Build history of the part. All positions in model axes, mm. Face numbers are marked on the shaded views. A direction names the side the tool comes from. Round coordinates to 2 decimals unless told otherwise and drop trailing zeros. Write each loop counter-clockwise with the first axis right and the second up, starting at its lowest first coordinate (ties: lowest second). Pieces come first, ordered by that corner, then holes. Notation, with made-up numbers: (-3.5, 19) -> (34.5, 19) arc R33 cw to (34.5, 58) -> close; hole circle Ø4 at (65.5, 49.5). An arc over 180 degrees is marked (long way). Answer as CSV lines item,"result".
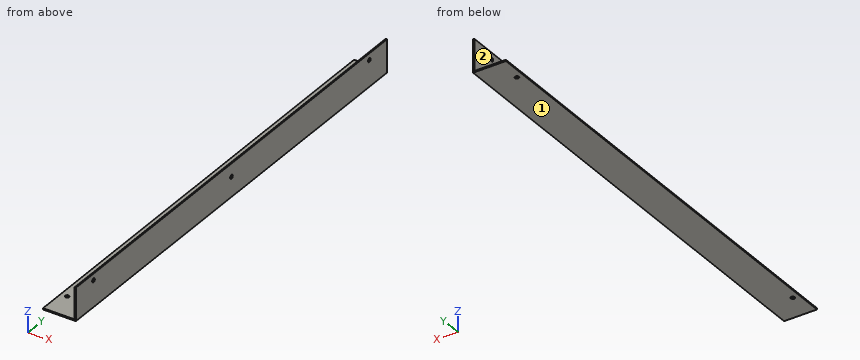
from build123d import *

# Parameters (mm, degrees)
CROQUIS2_W              = 1
CROQUIS2_H              = 354
SALIENTE_EXTRUIR2_DEPTH = 25
CROQUIS5_R              = 1.5
CORTAR_EXTRUIR2_DEPTH   = 1
CROQUIS1_W              = 24
CROQUIS1_H              = 354
CROQUIS1_R              = 1.5
SALIENTE_EXTRUIR3_DEPTH = 1


with BuildPart() as part:
    # Croquis2 → Saliente-Extruir2 (new body)
    with BuildSketch(Plane.XY):
        with Locations((-55.758230402, -111.819349421)):
            Rectangle(CROQUIS2_W, CROQUIS2_H)
    extrude(amount=SALIENTE_EXTRUIR2_DEPTH)

    # Croquis5 → Cortar-Extruir2 (cut)
    with BuildSketch(Plane(origin=(-55.258230402, 0, 0), x_dir=(0, 0, -1), z_dir=(1, 0, 0))):
        with Locations((-20, 45.180650579)):
            Circle(CROQUIS5_R)
        with Locations((-20, -268.819349421)):
            Circle(CROQUIS5_R)
        with Locations((-15, -111.819349421)):
            Circle(CROQUIS5_R)
    extrude(amount=-CORTAR_EXTRUIR2_DEPTH, mode=Mode.SUBTRACT)

    # Croquis1 → Saliente-Extruir3 (add)
    with BuildSketch(Plane.XY):
        with Locations((-68.258230402, -111.819349421)):
            Rectangle(CROQUIS1_W, CROQUIS1_H)
        with Locations((-75.258230402, 45.180650579)):
            Circle(CROQUIS1_R, mode=Mode.SUBTRACT)
        with Locations((-75.258230402, -268.819349421)):
            Circle(CROQUIS1_R, mode=Mode.SUBTRACT)
    extrude(amount=SALIENTE_EXTRUIR3_DEPTH)


solid = part.part
1. Which spindle directions (+Z, -Z, +X, -X, +Y, -Y) get a long thin tool onto all of the face, cutting with end or side? Do the marked faces 1 and 2. Say none if no direction does.
Results found:
face 1,"-Z, +X, -X, +Y, -Y"
face 2,"+Z, -X, +Y, -Y"
2. Cut at A-A, the plane y = -66. Write the cut outline in (x, z), then the cut area to 3 significant figures.
Results found:
outline,"(-80.26, 0) -> (-55.26, 0) -> (-55.26, 25) -> (-56.26, 25) -> (-56.26, 1) -> (-80.26, 1) -> close"
area,"49.0 mm2"
3. Probe line 1 along Z through (x, y) = (-71, -182); line 2 along X through (y, z) = (-236, 19.5); line 3 along Y through (x, z) = (-55.5, 15). List the from-to ranges inside material, lowest first.
Results found:
line 1,"z = 0 to 1"
line 2,"x = -56.26 to -55.26"
line 3,"y = -288.82 to -113.32, -110.32 to 65.18"
4. Cut at B-B, the plane z = 6.5. Write the cut outline in (x, y).
Results found:
outline,"(-56.26, -288.82) -> (-55.26, -288.82) -> (-55.26, 65.18) -> (-56.26, 65.18) -> close"
5. Drop flat-ended pins along their axis: pin 1 Ø1 at (x, y) = (-66, -203) entering from -Z; pin 2 Ø2 at (y, z) = (-29.5, 8) entering from -X; pin 3 Ø2.5 at (y, z) = (-268.82, 20) entering from +X; pin 4 Ø12 at (x, y) = (-65.5, -164.5) entering from +Z. Give the stop position or say it passes through.
Results found:
pin 1,"stops at z = 0"
pin 2,"stops at x = -56.26"
pin 3,"passes through"
pin 4,"stops at z = 1"
